Verification items for the finished model (mm, model axes). A direction names the side the tool comes from. Give positions to 0.01 mm unless a question says otherwise; leave off trailing zeros. Order: outer loops, then holes, each group sorted by start corner. A loop starts at its lowest first (then second) coordinate and runs counter-clockwise, first axis right, second up. Notation, with made-up numbers: (-12, -35.5) -> (27, -35.5) arc R18 cw to (27, -31.5) -> close; hole circle Ø5 at (29.5, 54.25). An arc over 180 degrees is marked (long way). Return JSON: item names as keys, results as strings. Group by question number.
(1) Release check for a two-part mould opening along Y. For faces 3 (the face through (1350, 3407.242, 9)), 4 (the face through (1428, 2759.242, 9)), 5 (the face through (1280.062, 3104, 9)) record: pulls with the +Y half, pulls with the -Y half, needs draft (parallel to the pull), parting line crosses it, or undercut.
(2) Tool access check on faces 1 (the face through (1510, 3105.242, 9)), 2 (the face through (1432, 3439.242, 9)). Record the directions out of +Z, -Z, +X, -X, +Y, -Y that give a thin tool (end or side, any length) a straight path to the whole face; none if there is none.
(3) Thickness scan on line 1 along Y through (x, z) = (1518, 15); line 2 along Y through (x, z) = (1369.5, 3.5); line 3 along X through (y, z) = (3411, 16.5). Record the ranges inside material, lowest first.
(4) Cross-section at A-A on x = 1518. Enter the section's corners in (y, z), then the cut area to 3 significant figures.
(5) Cross-section at B-B on z = 8. State how many separate pieces and enclosed holes the cut face has, then the cut area to 3 significant figures.
from build123d import *

# Parameters (mm, degrees)
BOSS_EXTRUDE1_DEPTH = 18


with BuildPart() as part:
    # Sketch1 → Boss-Extrude1 (new body)
    with BuildSketch(Plane.XY):
        Polygon((1280.062211089, 3439.241832817), (1280.062211089, 3419.241832817), (1280.062211089, 3407.241832817), (1280.062211089, 3105.241832817), (1280.062211089, 3093.241832817), (1280.062211089, 2791.241832817), (1280.062211089, 2779.241832817), (1280.062211089, 2759.241832817), (1580.062211089, 2759.241832817), (1580.062211089, 2779.241832817), (1580.062211089, 2791.241832817), (1580.062211089, 3093.241832817), (1580.062211089, 3105.241832817), (1580.062211089, 3407.241832817), (1580.062211089, 3419.241832817), (1580.062211089, 3439.241832817), align=None)
        with BuildLine():
            Line((1525.721822549, 3093.241832817), (1494.402599629, 3093.241832817))
            ThreePointArc((1494.402599629, 3093.241832817), (1489.178327612, 3092.357949341), (1490.062211089, 3097.582221357))
            Line((1490.062211089, 3097.582221357), (1490.062211089, 3100.901444277))
            ThreePointArc((1490.062211089, 3100.901444277), (1489.178327612, 3106.125716294), (1494.402599629, 3105.241832817))
            Line((1494.402599629, 3105.241832817), (1525.721822549, 3105.241832817))
            ThreePointArc((1525.721822549, 3105.241832817), (1530.946094565, 3106.125716294), (1530.062211089, 3100.901444277))
            Line((1530.062211089, 3100.901444277), (1530.062211089, 3097.582221357))
            ThreePointArc((1530.062211089, 3097.582221357), (1530.946094565, 3092.357949341), (1525.721822549, 3093.241832817))
        make_face(mode=Mode.SUBTRACT)
        with BuildLine():
            Line((1365.721822549, 2791.241832817), (1334.402599629, 2791.241832817))
            ThreePointArc((1334.402599629, 2791.241832817), (1329.178327612, 2792.125716294), (1330.062211089, 2786.901444277))
            Line((1330.062211089, 2786.901444277), (1330.062211089, 2783.582221357))
            ThreePointArc((1330.062211089, 2783.582221357), (1329.178327612, 2778.357949341), (1334.402599629, 2779.241832817))
            Line((1334.402599629, 2779.241832817), (1365.721822549, 2779.241832817))
            ThreePointArc((1365.721822549, 2779.241832817), (1370.946094565, 2778.357949341), (1370.062211089, 2783.582221357))
            Line((1370.062211089, 2783.582221357), (1370.062211089, 2786.901444277))
            ThreePointArc((1370.062211089, 2786.901444277), (1370.946094565, 2792.125716294), (1365.721822549, 2791.241832817))
        make_face(mode=Mode.SUBTRACT)
        with BuildLine():
            Line((1330.062211089, 3414.901444277), (1330.062211089, 3411.582221357))
            ThreePointArc((1330.062211089, 3411.582221357), (1329.178327612, 3406.357949341), (1334.402599629, 3407.241832817))
            Line((1334.402599629, 3407.241832817), (1365.721822549, 3407.241832817))
            ThreePointArc((1365.721822549, 3407.241832817), (1370.946094565, 3406.357949341), (1370.062211089, 3411.582221357))
            Line((1370.062211089, 3411.582221357), (1370.062211089, 3414.901444277))
            ThreePointArc((1370.062211089, 3414.901444277), (1370.946094565, 3420.125716294), (1365.721822549, 3419.241832817))
            Line((1365.721822549, 3419.241832817), (1334.402599629, 3419.241832817))
            ThreePointArc((1334.402599629, 3419.241832817), (1329.178327612, 3420.125716294), (1330.062211089, 3414.901444277))
        make_face(mode=Mode.SUBTRACT)
        with BuildLine():
            Line((1334.402599629, 3105.241832817), (1365.721822549, 3105.241832817))
            ThreePointArc((1365.721822549, 3105.241832817), (1370.946094565, 3106.125716294), (1370.062211089, 3100.901444277))
            Line((1370.062211089, 3100.901444277), (1370.062211089, 3097.582221357))
            ThreePointArc((1370.062211089, 3097.582221357), (1370.946094565, 3092.357949341), (1365.721822549, 3093.241832817))
            Line((1365.721822549, 3093.241832817), (1334.402599629, 3093.241832817))
            ThreePointArc((1334.402599629, 3093.241832817), (1329.178327612, 3092.357949341), (1330.062211089, 3097.582221357))
            Line((1330.062211089, 3097.582221357), (1330.062211089, 3100.901444277))
            ThreePointArc((1330.062211089, 3100.901444277), (1329.178327612, 3106.125716294), (1334.402599629, 3105.241832817))
        make_face(mode=Mode.SUBTRACT)
        with BuildLine():
            Line((1530.062211089, 2783.582221357), (1530.062211089, 2786.901444277))
            ThreePointArc((1530.062211089, 2786.901444277), (1530.946094565, 2792.125716294), (1525.721822549, 2791.241832817))
            Line((1525.721822549, 2791.241832817), (1494.402599629, 2791.241832817))
            ThreePointArc((1494.402599629, 2791.241832817), (1489.178327612, 2792.125716294), (1490.062211089, 2786.901444277))
            Line((1490.062211089, 2786.901444277), (1490.062211089, 2783.582221357))
            ThreePointArc((1490.062211089, 2783.582221357), (1489.178327612, 2778.357949341), (1494.402599629, 2779.241832817))
            Line((1494.402599629, 2779.241832817), (1525.721822549, 2779.241832817))
            ThreePointArc((1525.721822549, 2779.241832817), (1530.946094565, 2778.357949341), (1530.062211089, 2783.582221357))
        make_face(mode=Mode.SUBTRACT)
        with BuildLine():
            Line((1494.402599629, 3407.241832817), (1525.721822549, 3407.241832817))
            ThreePointArc((1525.721822549, 3407.241832817), (1530.946094565, 3406.357949341), (1530.062211089, 3411.582221357))
            Line((1530.062211089, 3411.582221357), (1530.062211089, 3414.901444277))
            ThreePointArc((1530.062211089, 3414.901444277), (1530.946094565, 3420.125716294), (1525.721822549, 3419.241832817))
            Line((1525.721822549, 3419.241832817), (1494.402599629, 3419.241832817))
            ThreePointArc((1494.402599629, 3419.241832817), (1489.178327612, 3420.125716294), (1490.062211089, 3414.901444277))
            Line((1490.062211089, 3414.901444277), (1490.062211089, 3411.582221357))
            ThreePointArc((1490.062211089, 3411.582221357), (1489.178327612, 3406.357949341), (1494.402599629, 3407.241832817))
        make_face(mode=Mode.SUBTRACT)
    extrude(amount=BOSS_EXTRUDE1_DEPTH)


solid = part.part
Verdict:
{
 "1": {"face 3": "undercut", "face 4": "pulls with the -Y half", "face 5": "needs draft"},
 "2": {"face 1": "+Z, -Z", "face 2": "+Z, -Z, +X, -X, +Y"},
 "3": {"line 1": "2759.24 to 2779.24, 2791.24 to 3093.24, 3105.24 to 3407.24, 3419.24 to 3439.24", "line 2": "2759.24 to 2777.52, 2792.96 to 3091.52, 3106.96 to 3405.52, 3420.96 to 3439.24", "line 3": "1280.06 to 1329.23, 1370.9 to 1489.23, 1530.9 to 1580.06"},
 "4": {"outline": "(2759.24, 0) -> (2779.24, 0) -> (2779.24, 18) -> (2759.24, 18) -> close; (2791.24, 0) -> (3093.24, 0) -> (3093.24, 18) -> (2791.24, 18) -> close; (3105.24, 0) -> (3407.24, 0) -> (3407.24, 18) -> (3105.24, 18) -> close; (3419.24, 0) -> (3439.24, 0) -> (3439.24, 18) -> (3419.24, 18) -> close", "area": "11,600 mm²"},
 "5": {"separate pieces": "1", "enclosed holes": "6", "area": "201,000 mm²"}
}
